Model file for the job. Use its own axes, mm. Coordinates: 2 decimals unless noted, no trailing zeros. Order: outer loops, then holes, each group sorted by start corner. A loop starts at its lowest first (then second) coordinate and runs counter-clockwise, first axis right, second up. Notation, with made-up numbers: M 1.25,-5 L 42.25,-5 A21 cw 42.25,2 Z; hole C -29.5,18 d5. An arc over 180 degrees is marked long. Return JSON: item names as keys, results as strings.
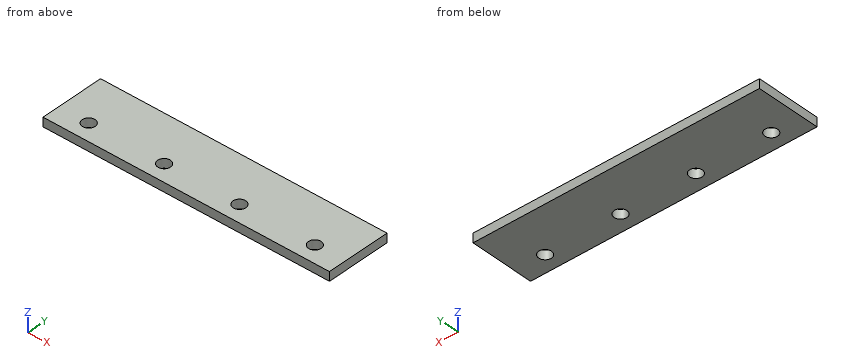
```python
from build123d import *

# Parameters (mm, degrees)
F0_W     = 190
F0_H     = 85
F0_R     = 8.5
F1_DEPTH = 12


with BuildPart() as f1:
    # F0 (on Top) → F1 (new body)
    with BuildSketch(Plane.XY):
        with Locations((95, 42.5)):
            Rectangle(F0_W, F0_H)
        with Locations((40, 23)):
            Circle(F0_R, mode=Mode.SUBTRACT)
        with Locations((140, 23)):
            Circle(F0_R, mode=Mode.SUBTRACT)
        with Locations((285, 42.5)):
            Rectangle(F0_W, F0_H)
        with Locations((240, 23)):
            Circle(F0_R, mode=Mode.SUBTRACT)
        with Locations((340, 23)):
            Circle(F0_R, mode=Mode.SUBTRACT)
    extrude(amount=F1_DEPTH)


solid = f1.part
```
Item 1: Drop a flat-ended pin along its axis: pin 1 Ø13.5 at (x, y) = (140, 23) entering from +Z. Give the stop position or say it passes through.
Check result:
{"pin 1": "passes through"}
Item 2: Wall check: line 1 (Y direction, x = 140, z = 5.75); line 2 (X direction, y = 30, z = 9.75). Give the ranges that are in metal, low to high.
Check result:
{"line 1": "y = 0 to 14.5, 31.5 to 85", "line 2": "x = 0 to 35.18, 44.82 to 135.18, 144.82 to 235.18, 244.82 to 335.18, 344.82 to 380"}
Item 3: Saw through at C-C (z = 2). Write the cut outline in (x, y), and give its area (3 significant figures).
Check result:
{"outline": "M 0,0 L 380,0 L 380,85 L 0,85 Z; hole C 40,23 d17; hole C 140,23 d17; hole C 240,23 d17; hole C 340,23 d17", "area": "31,400 mm2"}
Item 4: Saw through at A-A (x = 140). Write the cut outline in (y, z).
Check result:
{"outline": "M 0,0 L 14.5,0 L 14.5,12 L 0,12 Z; M 31.5,0 L 85,0 L 85,12 L 31.5,12 Z"}
Item 5: Saw through at B-B (y = 23). Write the cut outline in (x, z).
Check result:
{"outline": "M 0,0 L 31.5,0 L 31.5,12 L 0,12 Z; M 48.5,0 L 131.5,0 L 131.5,12 L 48.5,12 Z; M 148.5,0 L 231.5,0 L 231.5,12 L 148.5,12 Z; M 248.5,0 L 331.5,0 L 331.5,12 L 248.5,12 Z; M 348.5,0 L 380,0 L 380,12 L 348.5,12 Z"}
